Here's how the part is built. I have some questions about the finished solid (model axes, mm). Face numbers are marked on the shaded views. A direction names the side the tool comes from. Coordinates: 2 decimals unless noted, no trailing zeros. Write each loop counter-clockwise with the first axis right and the second up, starting at its lowest first coordinate (ties: lowest second). Pieces come first, ordered by that corner, then holes. Notation, with made-up numbers: M 73,39 L 87,39 A15 ccw 87,49 Z; hole C 86,51.5 d1. An arc over 180 degrees is marked long. Use one line per item in the form item = value. Start each with the question number.
1. I want a section at A-A, the plane z = 27.5. List the corners of the cut face in (x, y) for me.
2. Thinking about a two-plate mould opening in Y: for the marked faces 4, 5, 6 and 7, which applies, released by +Y, released by -Y, zero draft, split by the parting line, or undercut?
3. On a 3-axis mill with a long thin cutter (end or side, diameter ignored), from which of +Z, -Z, +X, -X, +Y, -Y can I reach the whole of each face in a straight line? I mean the marked faces 1, 2 and 3. Say none if no direction works.
4. I'm going to push a flat-ended pin straight in: pin 1 Ø11 at (y, z) = (-1.5, 30) entering from +X. Where does the tip first touch, or does it pass through?
5. I want a section at B-B, the plane x = 17. List the corners of the cut face in (y, z) for me.
6. I want a section at C-C, the plane y = -11.5. List the corners of the cut face in (x, z) for me.
7. Please list where these lines run through material, in increasing order: line 1 along X through (y, z) = (-6, 8); line 2 along Y through (x, z) = (9, 14.5); line 3 along Z through (x, y) = (2, -9.5). Write a range as [from, to].
8. I want a section at D-D, the plane x = 3. List the corners of the cut face in (y, z) for me, plus the area to 3 significant figures.
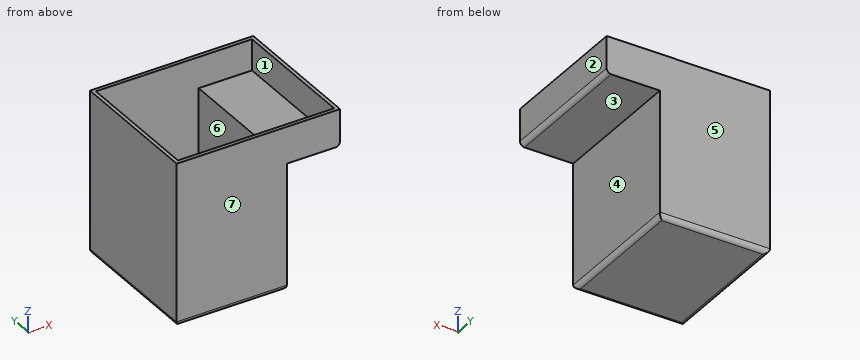
from build123d import *

# Parameters (mm, degrees)
F0_W     = 30.48
F0_H     = 38.1
F1_DEPTH = 1.524
F2_W     = 30.48
F2_H     = 38.1
F2_W_2   = 28.448
F2_H_2   = 36.068
F3_DEPTH = 33.274
F4_R     = 1.27
F5_W     = 45.212
F5_H     = 38.1
F5_W_2   = 28.448
F5_H_2   = 36.068
F6_DEPTH = 1.524
F7_W     = 45.212
F7_H     = 38.1
F7_W_2   = 43.18
F7_H_2   = 36.068
F8_DEPTH = 8.636
F9_R     = 1.27


with BuildPart() as f1:
    # F0 (on Top) → F1 (new body)
    with BuildSketch(Plane.XY):
        Rectangle(F0_W, F0_H)
    extrude(amount=F1_DEPTH)

    # F2 (on face) → F3 (join)
    with BuildSketch(Plane.XY.offset(1.524)):
        Rectangle(F2_W, F2_H)
        Rectangle(F2_W_2, F2_H_2, mode=Mode.SUBTRACT)
    extrude(amount=F3_DEPTH)

    # F4
    f4_edges = [f1.edges().sort_by_distance(p)[0] for p in [
        (0, 19.05, 0),
        (-15.24, 0, 0),
        (0, -19.05, 0),
        (15.24, 0, 0),
    ]]
    fillet(f4_edges, radius=F4_R)

    # F5 (on face) → F6 (join)
    with BuildSketch(Plane.XY.offset(34.798)):
        with Locations((7.366, 0)):
            Rectangle(F5_W, F5_H)
        Rectangle(F5_W_2, F5_H_2, mode=Mode.SUBTRACT)
    extrude(amount=F6_DEPTH)

    # F7 (on face) → F8 (join)
    with BuildSketch(Plane.XY.offset(36.322)):
        with Locations((7.366, 0)):
            Rectangle(F7_W, F7_H)
        with Locations((7.366, 0)):
            Rectangle(F7_W_2, F7_H_2, mode=Mode.SUBTRACT)
    extrude(amount=F8_DEPTH)

    # F9
    f9_edges = [f1.edges().sort_by_distance(p)[0] for p in [
        (29.972, 0, 34.798),
    ]]
    fillet(f9_edges, radius=F9_R)


solid = f1.part
Answer list:
q1.outline = M -15.24,-19.05 L 15.24,-19.05 L 15.24,19.05 L -15.24,19.05 Z; hole M -14.22,-18.03 L 14.22,-18.03 L 14.22,18.03 L -14.22,18.03 Z
q2.face_4 = zero draft
q2.face_5 = released by +Y
q2.face_6 = undercut
q2.face_7 = released by -Y
q3.face_1 = +Z
q3.face_2 = +Z, -Z, +X, +Y, -Y
q3.face_3 = -Z, +X, +Y, -Y
q4.pin_1 = 29.84
q5.outline = M -19.05,34.8 L 19.05,34.8 L 19.05,44.96 L 18.03,44.96 L 18.03,36.32 L -18.03,36.32 L -18.03,44.96 L -19.05,44.96 Z
q6.outline = M -15.24,1.27 A1.27 ccw -13.97,0 L 13.97,0 A1.27 ccw 15.24,1.27 L 15.24,34.8 L 28.7,34.8 A1.27 ccw 29.97,36.07 L 29.97,44.96 L 28.96,44.96 L 28.96,36.32 L 14.22,36.32 L 14.22,1.52 L -14.22,1.52 L -14.22,44.96 L -15.24,44.96 Z
q7.line_1 = [-15.24, -14.22], [14.22, 15.24]
q7.line_2 = [-19.05, -18.03], [18.03, 19.05]
q7.line_3 = [0, 1.52]
q8.outline = M -19.05,1.27 A1.27 ccw -17.78,0 L 17.78,0 A1.27 ccw 19.05,1.27 L 19.05,44.96 L 18.03,44.96 L 18.03,1.52 L -18.03,1.52 L -18.03,44.96 L -19.05,44.96 Z
q8.area = 146 mm²
